Verification items for the finished model (mm, model axes). Coordinates: 2 decimals unless noted, no trailing zeros. Loops run counter-clockwise (first coordinate to the right, second up) from the corner with the lowest first, then second, coordinate; pieces in that order, holes last. Notation, with made-up numbers: (89.5, 55.5) - (99.5, 55.5) arc R31 cw to (99.5, 87.5) - close; hole circle Ø11 at (2, -37.5). An arc over 180 degrees is marked (long way). One line per item, written item: value. Start each with the question number.
(1) Thickness scan on probe 1 along Y at (x, z) = (-52, -4); probe 2 along X at (y, z) = (-35, 22.5); probe 3 along Z at (x, y) = (-64, -24). Record the ranges inside material, lowest first. Write a range as [from, to].
(2) Draft check along Z on faces 1 (the face through (-50.28, -2.46, 36.3)), 2 (the face through (-43, -2, 44.739)), 3 (the face through (-60.774, -25, 32)). Enter one of: +Z half, -Z half, draft (parallel to the pull), parting line (faces both ways), or undercut.
(3) Section check C-C (z = 12). Record the boundary of the cut face in (x, y).
(4) Section check D-D (y = -3.5). Record the boundary of the cut face in (x, z).
(5) Gauge pin test, flat ends, axial feed: P1, Ø10, axis at x = -27, y = -8, coming from the -Z side; P2, Ø2.5, axis at x = -63, y = -28, coming from the +Z side; P3, Ø2.5, axis at y = -38.37, z = 34.69, coming from the -X side; P4, Ø4, axis at x = -51, z = -5.5, coming from the -Y side. Record the tip position at first contact, or that the pin passes through.
(6) Section check A-A (x = -47.5). Record the boundary of the cut face in (y, z), plus the area to 3 significant figures.
(7) Section check B-B (y = -16.5). Record the boundary of the cut face in (x, z).
```python
from build123d import *

# Parameters (mm, degrees)
F0_R          = 2.25
F1_DEPTH      = 5
F2_R          = 2.25
F3_DEPTH      = 5
F4_W          = 5
F4_H          = 55
F5_DEPTH      = 5
F6_W          = 25
F6_H          = 25
F7_DEPTH      = 5.195
F7_DEPTH_BACK = 35
F8_SIZE       = 5


with BuildPart() as f1:
    # F0 (on Front) → F1 (new body)
    with BuildSketch(Plane.XZ):
        Polygon((-20.774203624, 44.7394914553), (-60.774203624, 44.7394914553), (-60.774203624, 24.7394914553), (-60.774203624, -10.2605085447), (-40.774203624, -10.2605085447), (-20.774203624, 24.7394914553), align=None)
        with Locations((-48.619884952, 34.7818620503)):
            Circle(F0_R, mode=Mode.SUBTRACT)
        with Locations((-37.538797351, 34.7818620503)):
            Circle(F0_R, mode=Mode.SUBTRACT)
        with Locations((-26.3895275705, 34.7818620503)):
            Circle(F0_R, mode=Mode.SUBTRACT)
    extrude(amount=F1_DEPTH)



with BuildPart() as f3:
    # F2 (on face) → F3 (new body)
    with BuildSketch(Plane(origin=(-60.774203624, 0, 0), x_dir=(0, -1, 0), z_dir=(-1, 0, 0))):
        Polygon((44.9674582002, 44.6888683979), (5, 44.6888683979), (5, -10.2605085447), (4.9674582002, -10.2605085447), (4.9674582002, -10.3111316021), (24.9674582002, -10.3111316021), (44.9674582002, 24.6888683979), align=None)
        with Locations((16.1363705993, 34.6888683979)):
            Circle(F2_R, mode=Mode.SUBTRACT)
        with Locations((27.2174582002, 34.6888683979)):
            Circle(F2_R, mode=Mode.SUBTRACT)
        with Locations((38.3667279808, 34.6888683979)):
            Circle(F2_R, mode=Mode.SUBTRACT)
    extrude(amount=F3_DEPTH)


with BuildPart() as f1_1:
    add(f1.part)

    add(f3.part)  # F5 merges F3
    # F4 (on face) → F5 (join)
    with BuildSketch(Plane(origin=(-60.774203624, 0, 0), x_dir=(0, -1, 0), z_dir=(-1, 0, 0))):
        with Locations((2.5, 17.2394914553)):
            Rectangle(F4_W, F4_H)
    extrude(amount=F5_DEPTH)

    # F6 (on face) → F7 (join, two sides)
    with BuildSketch(Plane(origin=(0, 0, -10.2605085447), x_dir=(1, 0, 0), z_dir=(0, 0, -1))) as f7_sk:
        with Locations((-53.274203624, 12.5)):
            Rectangle(F6_W, F6_H)
    extrude(amount=F7_DEPTH)
    extrude(f7_sk.sketch, amount=-F7_DEPTH_BACK)

    # F8
    f8_edges = [f1_1.edges().sort_by_distance(p)[0] for p in [
        (-60.774204, -25, 7.242654),
        (-40.774204, -5, 7.239491),
    ]]
    chamfer(f8_edges, length=F8_SIZE)


solid = f1_1.part
```
Responses:
1. probe 1: y = [-25, 0]
1. probe 2: x = [-65.77, -60.77]
1. probe 3: z = [-15.46, 44.69]
2. face 1: undercut
2. face 2: +Z half
2. face 3: draft
3. outline: (-65.77, -37.72) - (-60.77, -37.72) - (-60.77, -30) - (-55.77, -25) - (-40.77, -25) - (-40.77, -10) - (-35.77, -5) - (-28.05, -5) - (-28.05, 0) - (-65.77, 0) - close
4. outline: (-65.77, -15.46) - (-40.77, -15.46) - (-40.77, -10.26) - (-20.77, 24.74) - (-20.77, 44.74) - (-65.77, 44.74) - close; hole circle Ø4.5 at (-48.62, 34.78); hole circle Ø4.5 at (-37.54, 34.78); hole circle Ø4.5 at (-26.39, 34.78)
5. P1: stops at z = 6.84
5. P2: stops at z = 44.69
5. P3: passes through
5. P4: stops at y = -25
6. outline: (-25, -15.46) - (0, -15.46) - (0, 32.83) - (-5, 32.83) - (-5, 24.74) - (-25, 24.74) - close; (-5, 36.73) - (0, 36.73) - (0, 44.74) - (-5, 44.74) - close
6. area: 1,090 mm²
7. outline: (-65.77, -15.46) - (-40.77, -15.46) - (-40.77, 24.74) - (-60.77, 24.74) - (-60.77, 32.47) - (-65.77, 32.47) - close; (-65.77, 36.91) - (-60.77, 36.91) - (-60.77, 44.69) - (-65.77, 44.69) - close
